```python
from build123d import *

# Parameters (mm, degrees)
SKETCH1_W           = 101.6
SKETCH1_H           = 101.6
BOSS_EXTRUDE1_DEPTH = 6.35
SKETCH2_W           = 6.35
SKETCH2_H           = 12.7
SKETCH2_H_2         = 6.35
CUT_EXTRUDE1_DEPTH  = 144.824345992
SKETCH2_3_W         = 6.35
SKETCH2_3_H         = 6.35
SKETCH2_3_W_2       = 12.7
CUT_EXTRUDE2_DEPTH  = 6.35


with BuildPart() as part:
    # Sketch1 → Boss-Extrude1 (new body)
    with BuildSketch(Plane(origin=(0, 0, 0), x_dir=(1, 0, 0), z_dir=(0, 1, 0))):
        with Locations((50.8, 50.8)):
            Rectangle(SKETCH1_W, SKETCH1_H)
    extrude(amount=BOSS_EXTRUDE1_DEPTH)

    # Sketch2 → Cut-Extrude1 (cut, through all)
    with BuildSketch(Plane(origin=(0, 6.35, 0), x_dir=(1, 0, 0), z_dir=(0, 1, 0))):
        with Locations((3.175, 82.55)):
            Rectangle(SKETCH2_W, SKETCH2_H)
        with Locations((3.175, 57.15)):
            Rectangle(SKETCH2_W, SKETCH2_H)
        with Locations((3.175, 31.75)):
            Rectangle(SKETCH2_W, SKETCH2_H)
        with Locations((3.175, 9.525)):
            Rectangle(SKETCH2_W, SKETCH2_H_2)
        with Locations((98.425, 95.25)):
            Rectangle(SKETCH2_W, SKETCH2_H)
        with Locations((98.425, 69.85)):
            Rectangle(SKETCH2_W, SKETCH2_H)
        with Locations((98.425, 44.45)):
            Rectangle(SKETCH2_W, SKETCH2_H)
        with Locations((98.425, 19.05)):
            Rectangle(SKETCH2_W, SKETCH2_H)
    extrude(amount=-CUT_EXTRUDE1_DEPTH, mode=Mode.SUBTRACT)

    # Sketch2_3 → Cut-Extrude2 (cut)
    with BuildSketch(Plane(origin=(0, 6.35, 0), x_dir=(1, 0, 0), z_dir=(0, 1, 0))):
        with Locations((9.525, 98.425)):
            Rectangle(SKETCH2_3_W, SKETCH2_3_H)
        with Locations((31.75, 98.425)):
            Rectangle(SKETCH2_3_W_2, SKETCH2_3_H)
        with Locations((57.15, 98.425)):
            Rectangle(SKETCH2_3_W_2, SKETCH2_3_H)
        with Locations((82.55, 98.425)):
            Rectangle(SKETCH2_3_W_2, SKETCH2_3_H)
        with Locations((82.55, 3.175)):
            Rectangle(SKETCH2_3_W_2, SKETCH2_3_H)
        with Locations((57.15, 3.175)):
            Rectangle(SKETCH2_3_W_2, SKETCH2_3_H)
        with Locations((31.75, 3.175)):
            Rectangle(SKETCH2_3_W_2, SKETCH2_3_H)
        with Locations((9.525, 3.175)):
            Rectangle(SKETCH2_3_W, SKETCH2_3_H)
        with Locations((3.175, 3.175)):
            Rectangle(SKETCH2_3_W, SKETCH2_3_H)
    extrude(amount=-CUT_EXTRUDE2_DEPTH, mode=Mode.SUBTRACT)


solid = part.part
```
For this review, take the finished solid that the model builds, in its own axes (mm). A direction names the side the tool comes from. Round coordinates to 2 decimals unless told otherwise and drop trailing zeros. Loops run counter-clockwise (first coordinate to the right, second up) from the corner with the lowest first, then second, coordinate; pieces in that order, holes last.
(1) We need section B-B (z = -91.5). Give the boundary of the cut face in (x, y), plus the area to 3 significant figures.
Returned:
outline: (0, 0) - (95.25, 0) - (95.25, 6.35) - (0, 6.35) - close
area: 605 mm2
(2) Mouldability with a two-part tool opening along X and no side actions: class faces 5 (the flat face through (38.1, 3, -98)), 6 (the flat face through (98, 3, -88.9)), 7 (the flat face through (0, 3, -44)) as released by +X, released by -X, zero draft, split by the parting line, or undercut.
Returned:
face 5: undercut
face 6: zero draft
face 7: released by -X
(3) Wall thickness on line 1 along X through (y, z) = (5, -14.5); line 2 along Z through (x, y) = (11, 3.25); line 3 along X through (y, z) = (2, -9.5): over which ranges is each line inside the solid? List them lowest first.
Returned:
line 1: x = 0 to 95.25
line 2: z = -95.25 to -6.35
line 3: x = 6.35 to 101.6
(4) We need section A-A (x = 58). Give the boundary of the cut face in (y, z), plus the area to 3 significant figures.
Returned:
outline: (0, -95.25) - (6.35, -95.25) - (6.35, -6.35) - (0, -6.35) - close
area: 565 mm2
(5) Clearance check with flat-ended pins moving along their axes: P1, Ø1.9, axis at y = 4, z = -99.5, coming from the +X side; P2, Ø1.9, axis at x = 100, y = 4.5, coming from the -Z side; P3, Ø1.9, axis at x = 83.5, y = 4, coming from the +Z side. State where each tip first meets the part, or that it passes through.
Returned:
P1: stops at x = 95.25
P2: stops at z = -88.9
P3: stops at z = -6.35
(6) Tool access review of faces 1 (the flat face through (3, 3, -63.5)), 2 (the flat face through (98, 3, -25.4)), 3 (the flat face through (25.4, 3, -3)), 4 (the flat face through (6.35, 3, -9)): name each direction out of +Z, -Z, +X, -X, +Y, -Y from which nothing blocks a thin tool from reaching the whole face with its end or side.
Returned:
face 1: -X, +Y, -Y
face 2: +X, +Y, -Y
face 3: +Z, +Y, -Y
face 4: +Z, -X, +Y, -Y
